Could you check a few things on this model? Use its own coordinates, in mm. Face numbers are marked on the shaded views. A direction names the side the tool comes from. Round coordinates to 2 decimals unless told otherwise and drop trailing zeros. Write each loop counter-clockwise with the first axis right and the second up, starting at its lowest first coordinate (ties: lowest second). Pieces come first, ordered by that corner, then holes. Notation, with made-up numbers: M 46.25,-4.5 L 101.25,-4.5 A15 cw 101.25,18.5 Z; hole C -36,33 d5. An arc over 180 degrees is marked long. One line per question, with ' | ' between items. Start each with the question number.
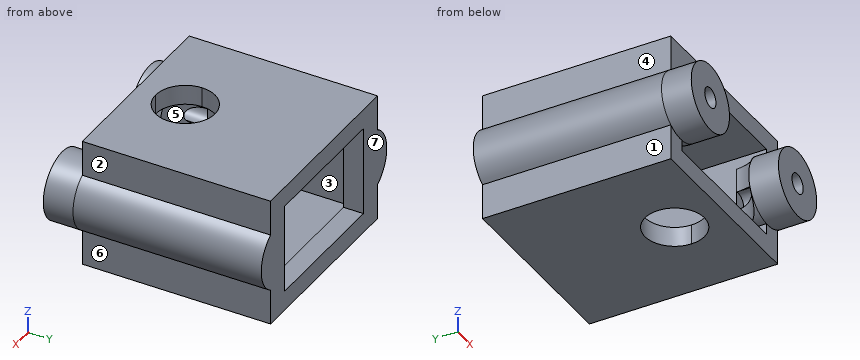
```python
from build123d import *

# Parameters (mm, degrees)
ESBO_O1_W                = 19
ESBO_O1_H                = 13
ESBO_O1_W_2              = 15
ESBO_O1_H_2              = 9
RESSALTO_EXTRUS_O1_DEPTH = 17
ESBO_O2_R                = 3.4
ESBO_O2_R_2              = 1
RESSALTO_EXTRUS_O2_DEPTH = 3
FILETE1_R                = 3
RESSALTO_EXTRUS_O3_START = 19
RESSALTO_EXTRUS_O3_DEPTH = 19
CORTE_EXTRUS_O1_DEPTH    = 26.579728302
ESBO_O5_W                = 0.5
ESBO_O5_H                = 1.584952831
ESBO_O5_W_2              = 2
ESBO_O5_H_2              = 5.830094338
RESSALTO_EXTRUS_O6_DEPTH = 2
CORTE_EXTRUS_O2_START    = -6
ESBO_O7_R                = 1
CORTE_EXTRUS_O2_DEPTH    = 6


with BuildPart() as part:
    # Esboço1 → Ressalto-extrusão1 (new body)
    with BuildSketch(Plane(origin=(0, 0, 0), x_dir=(1, 0, 0), z_dir=(0, 1, 0))):
        Rectangle(ESBO_O1_W, ESBO_O1_H)
        Rectangle(ESBO_O1_W_2, ESBO_O1_H_2, mode=Mode.SUBTRACT)
    extrude(amount=RESSALTO_EXTRUS_O1_DEPTH)

    # Esboço2 → Ressalto-extrusão2 (add)
    # profile 1 of 2: a face of its own
    with BuildSketch(Plane.XZ):
        with Locations(Location((7.75, 0, 0), (0, 0, 94.216730479))):
            Circle(ESBO_O2_R)
        with Locations(Location((7.75, 0, 0), (0, 0, 104.477512186))):
            Circle(ESBO_O2_R_2, mode=Mode.SUBTRACT)
    # profile 2 of 2: a face of its own
    with BuildSketch(Plane.XZ):
        with Locations(Location((-7.75, 0, 0), (0, 0, 85.783269521))):
            Circle(ESBO_O2_R)
        with Locations(Location((-7.75, 0, 0), (0, 0, 75.522487814))):
            Circle(ESBO_O2_R_2, mode=Mode.SUBTRACT)
    extrude(amount=RESSALTO_EXTRUS_O2_DEPTH)

    # Filete1
    # the kernel refuses this fillet: 3 mm, written as the material it adds along each edge
    with BuildSketch(Plane(origin=(-7.5, 0, -6.531754163), x_dir=(0, 1, 0), z_dir=(0, 0, 1))) as filete1_piece_1_section:
        with BuildLine():
            CenterArc((FILETE1_R, -FILETE1_R), FILETE1_R, 90, 90)
            Line((0, -FILETE1_R), (0, 0))
            Line((0, 0), (FILETE1_R, 0))
        make_face()
    filete1_piece_1 = extrude(amount=17.42255053, mode=Mode.PRIVATE)
    filete1_piece_1 = filete1_piece_1 & Plane(origin=(-7.75, 0.863183733, 0), x_dir=(0.07352941176727577, 0, 0.9972930490107501), z_dir=(0, 1, 0)) * Cylinder(3.4, 47, mode=Mode.PRIVATE)
    filete1_piece_1 = filete1_piece_1 - Plane(origin=(-7.75, 0.863183733, 0), x_dir=(0.25000000000118416, 0, 0.9682458365515485), z_dir=(0, 1, 0)) * Cylinder(1, 47, mode=Mode.PRIVATE)
    add(filete1_piece_1)
    with BuildSketch(Plane(origin=(-7.5, 0, -10.890796367), x_dir=(0, 1, 0), z_dir=(0, 0, 1))) as filete1_piece_2_section:
        with BuildLine():
            CenterArc((FILETE1_R, -FILETE1_R), FILETE1_R, 90, 90)
            Line((0, -FILETE1_R), (0, 0))
            Line((0, 0), (FILETE1_R, 0))
        make_face()
    filete1_piece_2 = extrude(amount=17.42255053, mode=Mode.PRIVATE)
    filete1_piece_2 = filete1_piece_2 & Plane(origin=(-7.75, 0.863183733, 0), x_dir=(0.07352941176727577, 0, 0.9972930490107501), z_dir=(0, 1, 0)) * Cylinder(3.4, 47, mode=Mode.PRIVATE)
    filete1_piece_2 = filete1_piece_2 - Plane(origin=(-7.75, 0.863183733, 0), x_dir=(0.25000000000118416, 0, 0.9682458365515485), z_dir=(0, 1, 0)) * Cylinder(1, 47, mode=Mode.PRIVATE)
    add(filete1_piece_2)
    with BuildSketch(Plane(origin=(7.5, 0, 6.531754163), x_dir=(0, 1, 0), z_dir=(0, 0, -1))) as filete1_piece_3_section:
        with BuildLine():
            CenterArc((FILETE1_R, -FILETE1_R), FILETE1_R, 90, 90)
            Line((0, -FILETE1_R), (0, 0))
            Line((0, 0), (FILETE1_R, 0))
        make_face()
    filete1_piece_3 = extrude(amount=17.42255053, mode=Mode.PRIVATE)
    filete1_piece_3 = filete1_piece_3 & Plane(origin=(7.75, 0.863183735, 0), x_dir=(-0.07352941176727565, 0, 0.9972930490107501), z_dir=(0, 1, 0)) * Cylinder(3.4, 47, mode=Mode.PRIVATE)
    filete1_piece_3 = filete1_piece_3 - Plane(origin=(7.75, 0.863183735, 0), x_dir=(-0.25000000000118405, 0, 0.9682458365515485), z_dir=(0, 1, 0)) * Cylinder(1, 47, mode=Mode.PRIVATE)
    add(filete1_piece_3)
    with BuildSketch(Plane(origin=(7.5, 0, 10.890796367), x_dir=(0, 1, 0), z_dir=(0, 0, -1))) as filete1_piece_4_section:
        with BuildLine():
            CenterArc((FILETE1_R, -FILETE1_R), FILETE1_R, 90, 90)
            Line((0, -FILETE1_R), (0, 0))
            Line((0, 0), (FILETE1_R, 0))
        make_face()
    filete1_piece_4 = extrude(amount=17.42255053, mode=Mode.PRIVATE)
    filete1_piece_4 = filete1_piece_4 & Plane(origin=(7.75, 0.863183735, 0), x_dir=(-0.07352941176727565, 0, 0.9972930490107501), z_dir=(0, 1, 0)) * Cylinder(3.4, 47, mode=Mode.PRIVATE)
    filete1_piece_4 = filete1_piece_4 - Plane(origin=(7.75, 0.863183735, 0), x_dir=(-0.25000000000118405, 0, 0.9682458365515485), z_dir=(0, 1, 0)) * Cylinder(1, 47, mode=Mode.PRIVATE)
    add(filete1_piece_4)

    # Esboço3 → Ressalto-extrusão3 (add)
    with BuildSketch(Plane(origin=(0, 0, 0), x_dir=(1, 0, 0), z_dir=(0, 1, 0)).offset(RESSALTO_EXTRUS_O3_START)):
        with BuildLine():
            Line((-9.5, -2.915047169), (-9.5, 2.915047169))
            ThreePointArc((-9.5, 2.915047169), (-11.15, 0), (-9.5, -2.915047169))
        make_face()
        with BuildLine():
            Line((9.5, 2.915047169), (9.5, -2.915047169))
            ThreePointArc((9.5, -2.915047169), (11.15, 0), (9.5, 2.915047169))
        make_face()
    extrude(amount=-RESSALTO_EXTRUS_O3_DEPTH)

    # Esboço6 → Corte-extrusão1 (cut, through all)
    with BuildSketch(Plane(origin=(0, 0, -6.5), x_dir=(-1, 0, 0), z_dir=(0, 0, -1))):
        with BuildLine():
            ThreePointArc((-3, 5), (-2.121320344, 2.878679656), (0, 2))
            Line((0, 2), (0, 5))
            Line((0, 5), (-3, 5))
        make_face()
        with BuildLine():
            Line((0, 5), (0, 2))
            ThreePointArc((0, 2), (2.121320344, 2.878679656), (3, 5))
            ThreePointArc((3, 5), (0, 8), (-3, 5))
            Line((-3, 5), (0, 5))
        make_face()
    extrude(amount=-CORTE_EXTRUS_O1_DEPTH, mode=Mode.SUBTRACT)

    # Esboço5 → Ressalto-extrusão6 (add)
    with BuildSketch(Plane(origin=(0, 17, 0), x_dir=(1, 0, 0), z_dir=(0, 1, 0))):
        Polygon((7.5, -4.5), (7, -4.5), (3, -4.5), (-3, -4.5), (-7, -4.5), (-7.5, -4.5), (-7.5, -2.915047169), (-9.5, -2.915047169), (-9.5, -6.5), (-3, -6.5), (3, -6.5), (9.5, -6.5), (9.5, -2.915047169), (7.5, -2.915047169), align=None)
        with Locations((7.25, -3.707523585)):
            Rectangle(ESBO_O5_W, ESBO_O5_H)
        with Locations((7.25, 3.707523585)):
            Rectangle(ESBO_O5_W, ESBO_O5_H)
        Polygon((3, 4.5), (7, 4.5), (7.5, 4.5), (7.5, 2.915047169), (9.5, 2.915047169), (9.5, 6.5), (3, 6.5), (-3, 6.5), (-9.5, 6.5), (-9.5, 2.915047169), (-7.5, 2.915047169), (-7.5, 4.5), (-7, 4.5), (-3, 4.5), align=None)
        with Locations((-7.25, -3.707523585)):
            Rectangle(ESBO_O5_W, ESBO_O5_H)
        with Locations((-7.25, 3.707523585)):
            Rectangle(ESBO_O5_W, ESBO_O5_H)
        with Locations((8.5, 0)):
            Rectangle(ESBO_O5_W_2, ESBO_O5_H_2)
        with Locations((-8.5, 0)):
            Rectangle(ESBO_O5_W_2, ESBO_O5_H_2)
        with Locations((-7.25, 0)):
            Rectangle(ESBO_O5_W, ESBO_O5_H_2)
        with Locations((7.25, 0)):
            Rectangle(ESBO_O5_W, ESBO_O5_H_2)
    extrude(amount=RESSALTO_EXTRUS_O6_DEPTH)

    # Esboço7 → Corte-extrusão2 (cut)
    with BuildSketch(Plane.XZ.offset(3).offset(CORTE_EXTRUS_O2_START)):
        with Locations(Location((-7.75, 0, 0), (0, 0, 75.522487814))):
            Circle(ESBO_O7_R)
        with Locations(Location((7.75, 0, 0), (0, 0, 104.477512186))):
            Circle(ESBO_O7_R)
    extrude(amount=CORTE_EXTRUS_O2_DEPTH, mode=Mode.SUBTRACT)


solid = part.part
```
1. Suppose I cut it at C-C (x = 1.25). Write out the boundary of the cut face in (y, z).
2. If we mould it in two halves opening along X, with no side actions, what happens to the marked faces 4, 5, 6 and 7? For each: released by +X, released by -X, zero draft, split by the parting line, or undercut.
3. I'm going to push flat-ended pins straight in: P1, Ø3, axis at y = 6, z = -5, coming from the -X side; P2, Ø1.8, axis at x = 3, z = 4.5, coming from the -Y side; P3, Ø1.6, axis at x = 7.75, z = 0, coming from the -Y side. Where does each tip first touch, or does it pass through?
4. Which directions (+Z, -Z, +X, -X, +Y, -Y) give clear straight access to the entire face, cutting with the end or side of a thin tool? Please do the marked faces 1, 2 and 3.
5. I need wall thicknesses on line 1 along X through (y, z) = (-0.55, 0); line 2 along X through (y, z) = (0.75, -3.5); line 3 along Z through (x, y) = (7.75, 1.7). Which ranges of each line are inside material? Lowest first, please. Write a range as from..to.
6. Suppose I cut it at A-A (z = -4). Write out the boundary of the cut face in (x, y).
7. Suppose I cut it at B-B (y = 10.75). Write out the boundary of the cut face in (x, z), and give its area (3 significant figures).
8. Suppose I cut it at D-D (y = 3.5). Write out the boundary of the cut face in (x, z).
Computed:
1) outline: M 0,-6.5 L 2.27,-6.5 L 2.27,-4.5 L 0,-4.5 Z; M 0,4.5 L 2.27,4.5 L 2.27,6.5 L 0,6.5 Z; M 7.73,-6.5 L 19,-6.5 L 19,-4.5 L 7.73,-4.5 Z; M 7.73,4.5 L 19,4.5 L 19,6.5 L 7.73,6.5 Z
2) face 4: released by -X | face 5: undercut | face 6: released by +X | face 7: zero draft
3) P1: stops at x = -9.5 | P2: stops at y = 0 | P3: stops at y = 3
4) face 1: -Z, -X, +Y, -Y | face 2: +Z, +X, +Y, -Y | face 3: none
5) line 1: x = -11.15..-8.75, -6.75..-4.35, 4.35..6.75, 8.75..11.15 | line 2: x = -9.5..-7.5, 7.5..9.5 | line 3: z = -6.5..-1, 1..6.5
6) outline: M -9.5,0 L -7.5,0 L -7.5,17 L -7,17 L -7,19 L -9.5,19 Z; M 7,17 L 7.5,17 L 7.5,0 L 9.5,0 L 9.5,19 L 7,19 Z
7) outline: M -9.5,-6.5 L 9.5,-6.5 L 9.5,-2.92 A3.4 ccw 9.5,2.92 L 9.5,6.5 L -9.5,6.5 L -9.5,2.92 A3.4 ccw -9.5,-2.92 Z; hole M -7.5,-4.5 L 7.5,-4.5 L 7.5,4.5 L -7.5,4.5 Z | area: 126 mm²
8) outline: M -9.5,-6.5 L -2.6,-6.5 L -2.6,-4.5 L -7.5,-4.5 L -7.5,4.5 L -2.6,4.5 L -2.6,6.5 L -9.5,6.5 L -9.5,2.92 A3.4 ccw -9.5,-2.92 Z; M 2.6,-6.5 L 9.5,-6.5 L 9.5,-2.92 A3.4 ccw 9.5,2.92 L 9.5,6.5 L 2.6,6.5 L 2.6,4.5 L 7.5,4.5 L 7.5,-4.5 L 2.6,-4.5 Z
